from build123d import *

# Parameters (mm, degrees)
SKETCH1_R           = 15
BOSS_EXTRUDE1_DEPTH = 4
SKETCH2_R           = 3.25
CUT_EXTRUDE1_DEPTH  = 3
SKETCH3_R           = 1.7
CUT_EXTRUDE2_DEPTH  = 22.587033145
SKETCH4_R           = 2
CUT_EXTRUDE3_DEPTH  = 2
SKETCH5_W           = 3
SKETCH5_H           = 15
BOSS_EXTRUDE2_DEPTH = 2
SKETCH7_W           = 1
SKETCH7_H           = 15
CUT_EXTRUDE4_DEPTH  = 1


with BuildPart() as part:
    # Sketch1 → Boss-Extrude1 (new body)
    with BuildSketch(Plane.XY):
        Circle(SKETCH1_R)
    extrude(amount=BOSS_EXTRUDE1_DEPTH)

    # Sketch2 → Cut-Extrude1 (cut)
    with BuildSketch(Plane(origin=(0, 0, 0), x_dir=(-1, 0, 0), z_dir=(0, 0, -1))):
        with Locations((-6.717514421, 6.717514421)):
            Circle(SKETCH2_R)
        with Locations((6.717514421, -6.717514421)):
            Circle(SKETCH2_R)
        with Locations((-5.656854249, -5.656854249)):
            Circle(SKETCH2_R)
        with Locations((5.656854249, 5.656854249)):
            Circle(SKETCH2_R)
    extrude(amount=-CUT_EXTRUDE1_DEPTH, mode=Mode.SUBTRACT)

    # Sketch3 → Cut-Extrude2 (cut, through all)
    with BuildSketch(Plane(origin=(0, 0, 0), x_dir=(-1, 0, 0), z_dir=(0, 0, -1))):
        with Locations((-6.717514421, 6.717514421)):
            Circle(SKETCH3_R)
        with Locations((5.656854249, 5.656854249)):
            Circle(SKETCH3_R)
        with Locations((6.717514421, -6.717514421)):
            Circle(SKETCH3_R)
        with Locations((-5.656854249, -5.656854249)):
            Circle(SKETCH3_R)
    extrude(amount=-CUT_EXTRUDE2_DEPTH, mode=Mode.SUBTRACT)

    # Sketch4 → Cut-Extrude3 (cut)
    with BuildSketch(Plane.XY.offset(3)):
        Circle(SKETCH4_R)
    extrude(amount=-CUT_EXTRUDE3_DEPTH, mode=Mode.SUBTRACT)

    # Sketch5 → Boss-Extrude2 (add)
    with BuildSketch(Plane.XY):
        Rectangle(SKETCH5_W, SKETCH5_H)
    extrude(amount=-BOSS_EXTRUDE2_DEPTH)

    # Sketch7 → Cut-Extrude4 (cut)
    with BuildSketch(Plane(origin=(0, 0, 0), x_dir=(-1, 0, 0), z_dir=(0, 0, -1))):
        with Locations((-1, 0)):
            Rectangle(SKETCH7_W, SKETCH7_H)
        with Locations((1, 0)):
            Rectangle(SKETCH7_W, SKETCH7_H)
    extrude(amount=CUT_EXTRUDE4_DEPTH, mode=Mode.SUBTRACT)


solid = part.part
Geometry: final body of the model. Coordinates: model frame, mm. A direction names the side the tool comes from. Coordinates: 2 decimals unless noted, no trailing zeros. Order: outer loops, then holes, each group sorted by start corner. A loop starts at its lowest first (then second) coordinate and runs counter-clockwise, first axis right, second up.
(1) Section query A-A (y = 0). Return the cut outline in (x, z), plus the area to 3 significant figures.
(2) Draft query along X for faces 5 (the face through (-14.985, 0.66, 1.972)), 6 (the face through (-8.1, -8.1, 3)), 7 (the face through (3, 0, 0)). Return one class per face: pulls with the +X half, pulls with the -X half, needs draft (parallel to the pull), parting line crosses it, or undercut.
(3) Material intervals for probe 1 along Y at (x, z) = (0, 2.05); probe 2 along X at (y, z) = (5.5, 2.55); probe 3 along X at (y, z) = (5.25, 2.4), sorted ascending.
(4) Section query B-B (x = -8). Return the cut outline in (y, z), plus the area to 3 significant figures.
(5) Section query D-D (z = 3.65). Return the cut outline in (x, y).
(6) First-contact query: pin 1 (2 mm diameter, centred on x = 5, z = 3, fed in from +Y); pin 2 (2 mm diameter, centred on y = -2, z = 0.5, fed in from +X); pin 3 (2.5 mm diameter, centred on x = -5.66, y = 5.66, fed in from -Z); pin 4 (6 mm diameter, centred on x = 5.66, y = -5.66, fed in from -Z). Flat tips, straight axial feed; report the tip coordinate or a pass-through.
(7) Section query C-C (x = 0). Return the cut outline in (y, z).
(8) Access query for faces 1 (the face through (0, -7.5, -1)), 2 (the face through (-0.5, -0.1, -0.5)), 3 (the face through (1, 0, -1)), 4 (the face through (-3.078, 3.679, 1.479)). Directions: +Z, -Z, +X, -X, +Y, -Y. A direction counts if a zero-diameter tool reaches every point of the face in a straight line with its end or side. Return the directions, or none.
Solution:
1. outline: (-15, 0) - (-0.5, 0) - (-0.5, -1) - (-1.5, -1) - (-1.5, -2) - (1.5, -2) - (1.5, -1) - (0.5, -1) - (0.5, 0) - (15, 0) - (15, 4) - (-15, 4) - close; hole (-2, 1) - (2, 1) - (2, 3) - (-2, 3) - close
1. area: 116 mm2
2. face 5: parting line crosses it
2. face 6: undercut
2. face 7: needs draft
3. probe 1: y = -15 to -2, 2 to 15
3. probe 2: x = -13.96 to -8.9, -2.41 to 3.7, 9.73 to 13.96
3. probe 3: x = -14.05 to -8.88, -2.43 to 3.82, 9.62 to 14.05
4. outline: (-12.69, 0) - (-9.7, 0) - (-9.7, 3) - (-7.83, 3) - (-7.83, 4) - (-12.69, 4) - close; (-5.6, 3) - (-3.73, 3) - (-3.73, 0) - (3.4, 0) - (3.4, 3) - (7.91, 3) - (7.91, 0) - (12.69, 0) - (12.69, 4) - (-5.6, 4) - close
4. area: 67.8 mm2
5. outline: circle Ø30 at (0, 0); hole circle Ø3.4 at (-6.72, -6.72); hole circle Ø3.4 at (-5.66, 5.66); hole circle Ø3.4 at (5.66, -5.66); hole circle Ø3.4 at (6.72, 6.72)
6. pin 1: stops at y = 14.46
6. pin 2: stops at x = 14.97
6. pin 3: passes through
6. pin 4: stops at z = 3
7. outline: (-15, 0) - (-7.5, 0) - (-7.5, -2) - (7.5, -2) - (7.5, 0) - (15, 0) - (15, 4) - (-15, 4) - close; hole (-2, 1) - (2, 1) - (2, 3) - (-2, 3) - close
8. face 1: -Z, +X, -X, -Y
8. face 2: -X, +Y, -Y
8. face 3: +X, +Y, -Y
8. face 4: -Z
